```python
from build123d import *

# Parameters (mm, degrees)
SKETCH1_W           = 25
SKETCH1_H           = 60
BOSS_EXTRUDE1_DEPTH = 30
SKETCH2_W           = 60
SKETCH2_H           = 8.623813306
BOSS_EXTRUDE2_DEPTH = 20
SKETCH3_R           = 4
CUT_EXTRUDE1_DEPTH  = 9.623813306
CUT_EXTRUDE2_DEPTH  = 20
BOSS_EXTRUDE3_DEPTH = 1


with BuildPart() as part:
    # Sketch1 → Boss-Extrude1 (new body)
    with BuildSketch(Plane(origin=(0, 0, 0), x_dir=(1, 0, 0), z_dir=(0, 1, 0))):
        Rectangle(SKETCH1_W, SKETCH1_H)
    extrude(amount=BOSS_EXTRUDE1_DEPTH)

    # Sketch2 → Boss-Extrude2 (add)
    with BuildSketch(Plane.ZY.offset(12.5)):
        with Locations((0, 4.311906653)):
            Rectangle(SKETCH2_W, SKETCH2_H)
    extrude(amount=BOSS_EXTRUDE2_DEPTH)

    # Sketch3 → Cut-Extrude1 (cut, through all)
    with BuildSketch(Plane(origin=(0, 8.623813306, 0), x_dir=(1, 0, 0), z_dir=(0, 1, 0))):
        with Locations(Location((-24.5, 20, 0), (0, 0, 270))):  # turned: the seam where the file's is
            Circle(SKETCH3_R)
        with Locations(Location((-24.5, -20, 0), (0, 0, 270))):  # turned: the seam where the file's is
            Circle(SKETCH3_R)
    extrude(amount=-CUT_EXTRUDE1_DEPTH, mode=Mode.SUBTRACT)

    # Sketch4 → Cut-Extrude2 (cut)
    with BuildSketch(Plane(origin=(12.5, 0, 0), x_dir=(0, 0, -1), z_dir=(1, 0, 0))):
        Polygon((-17.585328198, 3.984734315), (-4.601018482, 19.458832066), (-12.414671802, 26.015265685), (-25.398981518, 10.541167934), align=None)
    extrude(amount=-CUT_EXTRUDE2_DEPTH, mode=Mode.SUBTRACT)

    # Sketch5 → Boss-Extrude3 (add)
    with BuildSketch(Plane(origin=(0, 30, 0), x_dir=(1, 0, 0), z_dir=(0, 1, 0))):
        Polygon((-5.384615385, -10), (-5.384615385, 10), (-2.564102564, 10), (-2.564102564, -7.692307692), (6.923076923, -7.692307692), (6.923076923, -10), align=None)
    extrude(amount=BOSS_EXTRUDE3_DEPTH)


solid = part.part
```
The model under review builds one solid part; all positions refer to its coordinate system, in mm. A direction names the side the tool comes from. Round coordinates to 2 decimals unless told otherwise and drop trailing zeros. Write each loop counter-clockwise with the first axis right and the second up, starting at its lowest first coordinate (ties: lowest second). Pieces come first, ordered by that corner, then holes. Notation, with made-up numbers: (-29, -29.75) - (-16, -29.75) arc R34 cw to (-16, 0.25) - close; hole circle Ø1 at (-36.75, 55). An arc over 180 degrees is marked (long way). Use one line per item in the form item = value.
Q1. Tool access review of faces 5 (the flat face through (2.64, 22.69, 8.45)), 6 (the flat face through (12.5, 15, 0)): name each direction out of +Z, -Z, +X, -X, +Y, -Y from which nothing blocks a thin tool from reaching the whole face with its end or side.
Answer key:
face_5 = +X
face_6 = +Z, -Z, +X, +Y, -Y
Q2. Insertion check: pin 1 Ø5 at (x, z) = (-24.5, 20) entering from -Y; pin 2 Ø17 at (y, z) = (24.5, -7) entering from -X; pin 3 Ø13 at (x, z) = (-24.5, -20) entering from +Y; pin 4 Ø0.8 at (x, y) = (4, 30.5) entering from -Z. Each pin has a flat end and moves straight along its axis. Give the tip position at first contact, or say it passes through.
Answer key:
pin_1 = through
pin_2 = -12.5
pin_3 = 8.62
pin_4 = 7.69
Q3. Consider section C-C (z = -20). State the section outline as (x, y) points.
Answer key:
outline = (-32.5, 0) - (-28.5, 0) - (-28.5, 8.62) - (-32.5, 8.62) - close; (-20.5, 0) - (12.5, 0) - (12.5, 30) - (-12.5, 30) - (-12.5, 8.62) - (-20.5, 8.62) - close
Q4. For line 1 (X direction, y = 3.25, z = 20); line 2 (Z direction, x = -24, y = 6); line 3 (Y direction, x = -5, z = -14.5), list the stretches that pass through material, from the lowest coordinate up. Write a range as [from, to].
Answer key:
line_1 = [-32.5, -28.5], [-20.5, 12.5]
line_2 = [-30, -23.97], [-16.03, 16.03], [23.97, 30]
line_3 = [0, 30]
Q5. Draft analysis for pull direction X (two halves, no side actions). For faces 1 (the cylindrical face through (-20.534, 4.372, 19.479)), 2 (the cylindrical face through (-20.534, 4.372, -20.521)), 3 (the flat face through (-12.5, 19, 0)), 4 (the flat face through (-22, 8.624, 0)), state which applies: +X half, -X half, draft (parallel to the pull), parting line (faces both ways), or undercut.
Answer key:
face_1 = undercut
face_2 = undercut
face_3 = -X half
face_4 = draft
Q6. Consider section B-B (z = -1). State the section outline as (x, y) points.
Answer key:
outline = (-32.5, 0) - (12.5, 0) - (12.5, 30) - (-2.56, 30) - (-2.56, 31) - (-5.38, 31) - (-5.38, 30) - (-12.5, 30) - (-12.5, 8.62) - (-32.5, 8.62) - close
Q7. Consider section D-D (x = -24.5). State the section outline as (y, z) points.
Answer key:
outline = (0, -30) - (8.62, -30) - (8.62, -24) - (0, -24) - close; (0, -16) - (8.62, -16) - (8.62, 16) - (0, 16) - close; (0, 24) - (8.62, 24) - (8.62, 30) - (0, 30) - close
Q8. Consider section A-A (x = 9). State the section outline as (y, z) points, and give its area (3 significant figures).
Answer key:
outline = (0, -30) - (30, -30) - (30, 30) - (0, 30) - close; hole (3.98, 17.59) - (19.46, 4.6) - (26.02, 12.41) - (10.54, 25.4) - close
area = 1,590 mm2
